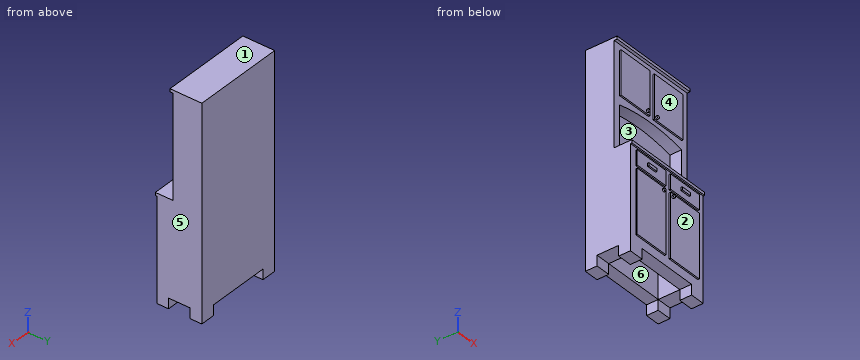
from build123d import *

# Parameters (mm, degrees)
F0_W      = 793.75
F0_H      = 402.59
F1_DEPTH  = 1828.8
F2_W      = 539.75
F2_H      = 88.9
F3_DEPTH  = 402.591
F2_W_2    = 312.801
F2_H_2    = 546.1
F2_H_3    = 127
F4_DEPTH  = 12.7
F2_H_4    = 374.65
F2_W_3    = 676.402
F2_H_5    = 387.35
F5_DEPTH  = 152.4
F6_DEPTH  = 254
F7_W      = 312.801
F7_H      = 374.65
F8_DEPTH  = 12.7
F9_W      = 186.69
F9_H      = 88.9
F10_DEPTH = 793.751
F11_W     = 88.9
F11_H     = 25.4
F11_R     = 12.7
F12_DEPTH = 12.7
F13_R     = 12.7
F14_DEPTH = 12.7
F15_W     = 793.75
F15_H     = 250.19
F15_H_2   = 25.4
F16_DEPTH = 25.4
F17_W     = 539.75
F17_H     = 186.69
F18_DEPTH = 609.6


with BuildPart() as f1:
    # F0 (on Top) → F1 (new body)
    with BuildSketch(Plane.XY):
        Rectangle(F0_W, F0_H)
    extrude(amount=F1_DEPTH)

    # F2 (on face) → F3 (cut, through all)
    with BuildSketch(Plane.XZ.offset(201.295)):
        with Locations((0, 44.45)):
            Rectangle(F2_W, F2_H)
    extrude(amount=-F3_DEPTH, mode=Mode.SUBTRACT)

    # F2 (on face) → F4 (cut)
    with BuildSketch(Plane.XZ.offset(201.295)):
        Polygon((-396.875, 0), (-269.875, 0), (-269.875, 88.9), (269.875, 88.9), (269.875, 0), (396.875, 0), (396.875, 889), (-396.875, 889), align=None)
        with Locations((-181.8005, 438.15)):
            Rectangle(F2_W_2, F2_H_2, mode=Mode.SUBTRACT)
        with Locations((-181.8005, 800.1)):
            Rectangle(F2_W_2, F2_H_3, mode=Mode.SUBTRACT)
        with Locations((181.8005, 438.15)):
            Rectangle(F2_W_2, F2_H_2, mode=Mode.SUBTRACT)
        with Locations((181.8005, 800.1)):
            Rectangle(F2_W_2, F2_H_3, mode=Mode.SUBTRACT)
    extrude(amount=-F4_DEPTH, mode=Mode.SUBTRACT)

    # F2 (on face) → F5 (cut)
    with BuildSketch(Plane.XZ.offset(201.295)):
        with BuildLine():
            Line((-396.875, 1828.8), (-396.875, 914.4))
            Line((-396.875, 914.4), (-338.201, 914.4))
            Line((-338.201, 914.4), (-338.201, 1301.75))
            ThreePointArc((-338.201, 1301.75), (0, 1339.749972), (338.201, 1301.75))
            Line((338.201, 1301.75), (338.201, 914.4))
            Line((338.201, 914.4), (396.875, 914.4))
            Line((396.875, 914.4), (396.875, 1828.8))
            Line((396.875, 1828.8), (-396.875, 1828.8))
        make_face()
        with Locations((-181.8005, 1565.275)):
            Rectangle(F2_W_2, F2_H_4, mode=Mode.SUBTRACT)
        with Locations((181.8005, 1565.275)):
            Rectangle(F2_W_2, F2_H_4, mode=Mode.SUBTRACT)
        with Locations((-181.8005, 1565.275)):
            Rectangle(F2_W_2, F2_H_4)
        with Locations((181.8005, 1565.275)):
            Rectangle(F2_W_2, F2_H_4)
        with Locations((0, 1108.075)):
            Rectangle(F2_W_3, F2_H_5)
    extrude(amount=-F5_DEPTH, mode=Mode.SUBTRACT)

    # F2 (on face) → F6 (cut)
    with BuildSketch(Plane.XZ.offset(201.295)):
        with Locations((0, 1108.075)):
            Rectangle(F2_W_3, F2_H_5)
        with BuildLine():
            ThreePointArc((338.201, 1301.75), (0, 1339.749972), (-338.201, 1301.75))
            Line((-338.201, 1301.75), (338.201, 1301.75))
        make_face()
    extrude(amount=-F6_DEPTH, mode=Mode.SUBTRACT)

    # F7 (on face) → F8 (join)
    with BuildSketch(Plane.XZ.offset(48.895)):
        with Locations((181.8005, 1565.275)):
            Rectangle(F7_W, F7_H)
        with Locations((-181.8005, 1565.275)):
            Rectangle(F7_W, F7_H)
    extrude(amount=F8_DEPTH)

    # F9 (on face) → F10 (cut, through all)
    with BuildSketch(Plane.YZ.offset(396.875)):
        with Locations((6.35, 44.45)):
            Rectangle(F9_W, F9_H)
    extrude(amount=-F10_DEPTH, mode=Mode.SUBTRACT)

    # F11 (on face) → F12 (join)
    with BuildSketch(Plane.XZ.offset(201.295)):
        with Locations((181.7116, 800.1)):
            Rectangle(F11_W, F11_H)
        with Locations((50.8, 685.8)):
            Circle(F11_R)
        with Locations((-50.8, 685.8)):
            Circle(F11_R)
        with Locations((-181.8005, 800.1)):
            Rectangle(F11_W, F11_H)
    extrude(amount=F12_DEPTH)

    # F13 (on face) → F14 (join)
    with BuildSketch(Plane.XZ.offset(61.595)):
        with Locations((-50.8, 1403.35)):
            Circle(F13_R)
        with Locations((50.8, 1403.35)):
            Circle(F13_R)
    extrude(amount=F14_DEPTH)

    # F15 (on face) → F16 (join)
    with BuildSketch(Plane.XY.offset(1828.8)):
        with Locations((0, 76.2)):
            Rectangle(F15_W, F15_H)
        with Locations((0, -61.595)):
            Rectangle(F15_W, F15_H_2)
    extrude(amount=-F16_DEPTH)

    # F17 (on face) → F18 (cut)
    with BuildSketch(Plane(origin=(0, 0, 88.9), x_dir=(1, 0, 0), z_dir=(0, 0, -1))):
        with Locations((0, -6.35)):
            Rectangle(F17_W, F17_H)
    extrude(amount=-F18_DEPTH, mode=Mode.SUBTRACT)


solid = f1.part
CAD build for the part. Positions are in the model's coordinates, mm. Face numbers are marked on the shaded views. A direction names the side the tool comes from. Round coordinates to 2 decimals unless told otherwise and drop trailing zeros. Write each loop counter-clockwise with the first axis right and the second up, starting at its lowest first coordinate (ties: lowest second). Pieces come first, ordered by that corner, then holes.
(1) Slice it at C-C, the plane z = 112.5. Write the cut outline in (x, y) (3 decimals), and give its area (3 significant figures).
(2) Slice it at D-D, the plane y = 144.5. Write the cut outline in (x, z) (3 decimals), and give its area (3 significant figures).
(3) Mould opens along Z. For the marked faces 1, 2, 3 and 4 say: pulls with the +Z half, pulls with the -Z half, needs draft (parallel to the pull), parting line crosses it, or undercut.
(4) Drop flat-ended pins along their axis: P1, Ø14, axis at x = -199.5, y = -205, coming from the +Z side; P2, Ø3, axis at x = 221, y = -28.5, coming from the -Z side; P3, Ø6.5, axis at x = 178, y = -209.5, coming from the -Z side. Give the stop position or say it passes through.
(5) Slice it at B-B, the plane z = 1648.5. Write the cut outline in (x, y) (3 decimals), and give its area (3 significant figures).
(6) Probe line 1 along Z through (x, y) = (-168.5, -49); line 2 along X through (y, z) = (0, 480) (3 decimals); line 3 along X through (y, z) = (9, 1231.5) (3 decimals). List the from-to ranges inside material, lowest first.
(7) 3-axis set-ups, long thin cutter, end or side, ignore diameter. For the marked faces 5 and 6: which of +Z, -Z, +X, -X, +Y, -Y reach the whole face in a straight line?
(8) Slice it at A-A, the plane y = -30. Write the cut outline in (x, z) (3 decimals).
From the geometry:
1. outline: (-396.875, -188.595) - (396.875, -188.595) - (396.875, 201.295) - (-396.875, 201.295) - close; hole (-269.875, -86.995) - (269.875, -86.995) - (269.875, 99.695) - (-269.875, 99.695) - close
1. area: 209,000 mm2
2. outline: (-396.875, 0) - (-269.875, 0) - (-269.875, 88.9) - (269.875, 88.9) - (269.875, 0) - (396.875, 0) - (396.875, 1828.8) - (-396.875, 1828.8) - close
2. area: 1,400,000 mm2
3. face 1: pulls with the +Z half
3. face 2: needs draft
3. face 3: undercut
3. face 4: undercut
4. P1: stops at z = 914.4
4. P2: stops at z = 698.5
4. P3: stops at z = 787.4
5. outline: (-396.875, -48.895) - (-338.201, -48.895) - (-338.201, -61.595) - (-25.4, -61.595) - (-25.4, -48.895) - (25.4, -48.895) - (25.4, -61.595) - (338.201, -61.595) - (338.201, -48.895) - (396.875, -48.895) - (396.875, 201.295) - (-396.875, 201.295) - close
5. area: 207,000 mm2
6. line 1: z = 698.5 to 914.4, 1377.95 to 1752.6, 1803.4 to 1828.8
6. line 2: x = -396.875 to -269.875, 269.875 to 396.875
6. line 3: x = -396.875 to -338.201, 338.201 to 396.875
7. face 5: +Z, -Z, +X, +Y, -Y
7. face 6: -Z
8. outline: (-396.875, 88.9) - (-269.875, 88.9) - (-269.875, 698.5) - (269.875, 698.5) - (269.875, 88.9) - (396.875, 88.9) - (396.875, 1828.8) - (-396.875, 1828.8) - close; hole (-338.201, 914.4) - (338.201, 914.4) - (338.201, 1301.75) arc R1524 ccw to (-338.201, 1301.75) - close
